Can you work these out from the drawing? Everything is in mm from the part's minimum corner. A direction names the side the tool comes from. Round coordinates to 2 decimals unless told otherwise and drop trailing zeros. Loops run counter-clockwise (first coordinate to the right, second up) from the corner with the lowest first, then second, coordinate; pieces in that order, holes last. Notation, with made-up numbers: M -33,70.25 L -2,70.25 A25 cw -2,105.25 Z; hole C 47,-30.75 d6. An arc over 180 degrees is marked long. Use a Markdown table: item, result.
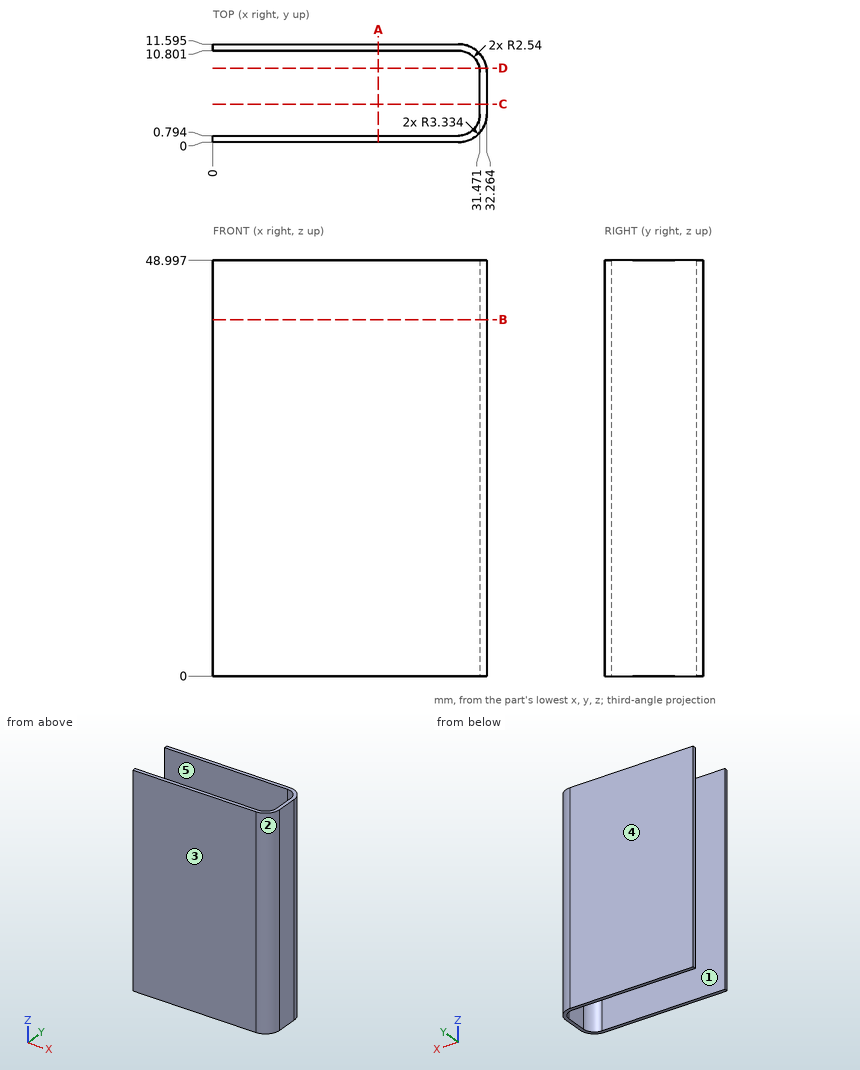
Q1. For the marked faces 1 and 2, which set-ups out of +Z, -Z, +X, -X, +Y, -Y let a thin tool reach every point of the face, with its end or its side?
Return value:
| item | result |
|---|---|
| face 1 | +Z, -Z, -X |
| face 2 | +Z, -Z, +X, -Y |
Q2. Imagine slicing it at A-A, the plane x = 19.5. Please give me the cut outline in (y, z) (1 decimal).
Return value:
| item | result |
|---|---|
| outline | M 0,0 L 0.8,0 L 0.8,49 L 0,49 Z; M 10.8,0 L 11.6,0 L 11.6,49 L 10.8,49 Z |
Q3. Imagine slicing it at B-B, the plane z = 42. Please give me the cut outline in (x, y) (1 decimal).
Return value:
| item | result |
|---|---|
| outline | M 0,0 L 28.9,0 A3.3 ccw 32.3,3.3 L 32.3,8.3 A3.3 ccw 28.9,11.6 L 0,11.6 L 0,10.8 L 28.9,10.8 A2.5 cw 31.5,8.3 L 31.5,3.3 A2.5 cw 28.9,0.8 L 0,0.8 Z |
Q4. I need wall thicknesses on line 1 (Y direction, x = 20, z = 23) (1 decimal); line 2 (X direction, y = 3.25, z = 14.5); line 3 (Y direction, x = 30.5, z = 6) (1 decimal). Which ranges of each line are inside material? Lowest first, please. Write a range as from..to.
Return value:
| item | result |
|---|---|
| line 1 | y = 0..0.8, 10.8..11.6 |
| line 2 | x = 31.47..32.26 |
| line 3 | y = 0.4..1.3, 10.3..11.2 |
Q5. Will these pins go through, and if not, where does the flat tip stop? P1, Ø1.5, axis at y = 6.5, z = 7.5, coming from the -X side; P2, Ø1.5, axis at x = 9, y = 9, coming from the +Z side.
Return value:
| item | result |
|---|---|
| P1 | stops at x = 31.47 |
| P2 | passes through |
Q6. Imagine slicing it at C-C, the plane y = 4.5. Please give me the cut outline in (x, z) (1 decimal).
Return value:
| item | result |
|---|---|
| outline | M 31.5,0 L 32.3,0 L 32.3,49 L 31.5,49 Z |
Q7. We'd pull the mould along Y, two halves only. Please class the marked faces 3, 4 and 5: pulls with the +Y half, pulls with the -Y half, needs draft (parallel to the pull), parting line crosses it, or undercut.
Return value:
| item | result |
|---|---|
| face 3 | pulls with the -Y half |
| face 4 | pulls with the +Y half |
| face 5 | undercut |
Q8. Imagine slicing it at D-D, the plane y = 8.75. Please give me the cut outline in (x, z).
Return value:
| item | result |
|---|---|
| outline | M 31.42,0 L 32.23,0 L 32.23,49 L 31.42,49 Z |
